Check sheet for the modelled part. Datum: model origin and axes. Units: mm. A direction names the side the tool comes from. Round coordinates to 2 decimals unless told otherwise and drop trailing zeros. Loops run counter-clockwise (first coordinate to the right, second up) from the corner with the lowest first, then second, coordinate; pieces in that order, holes last. Notation, with made-up numbers: (-24, 81) -> (-10, 81) arc R16 ccw to (-10, 87) -> close; hole circle Ø2 at (40, 53.25). An arc over 180 degrees is marked (long way). One line per question, with ' | ' between items.
```python
from build123d import *

# Parameters (mm, degrees)
BASE_EXTRUDE_DEPTH = 3


with BuildPart() as part:
    # Sketch1 → Base-Extrude (new body)
    with BuildSketch(Plane.XY):
        with BuildLine():
            Line((457.287518249, -79.214649933), (453.745445311, -79.230530857))
            ThreePointArc((453.745445311, -79.230530857), (449.646042877, -88.708611573), (453.753998991, -98.182988118))
            Line((453.753998991, -98.182988118), (469.771556658, -98.182988118))
            Line((469.771556658, -98.182988118), (469.765330169, -116.15983969))
            Line((469.765330169, -116.15983969), (483.771556658, -116.15983969))
            Line((483.771556658, -116.15983969), (483.771556658, -98.182988118))
            Line((483.771556658, -98.182988118), (485.771556658, -98.182988118))
            Line((485.771556658, -98.182988118), (485.434474546, -91.751078274))
            Line((485.434474546, -91.751078274), (488.434474546, -91.751078274))
            Line((488.434474546, -91.751078274), (488.771556658, -98.182988118))
            Line((488.771556658, -98.182988118), (499.789114325, -98.182988118))
            ThreePointArc((499.789114325, -98.182988118), (503.897070438, -88.708611573), (499.797668004, -79.230530857))
            Line((499.797668004, -79.230530857), (496.255595066, -79.214649933))
            Line((496.255595066, -79.214649933), (496.255595066, -91.387236838))
            Line((496.255595066, -91.387236838), (493.156556658, -91.387236838))
            Line((493.156556658, -91.387236838), (493.156556658, -81.698972351))
            Line((493.156556658, -81.698972351), (460.386556658, -81.698972351))
            Line((460.386556658, -81.698972351), (460.386556658, -91.387236838))
            Line((460.386556658, -91.387236838), (457.287518249, -91.387236838))
            Line((457.287518249, -91.387236838), (457.287518249, -79.214649933))
        make_face()
    extrude(amount=BASE_EXTRUDE_DEPTH)


solid = part.part
```
(1) Mould release check, pull along Y, two halves, no side actions. Record for faces 1 (the face through (485, -98.183, 1)), 2 (the face through (483.772, -107, 1)), 3 (the face through (485.605, -95.012, 1.479)): +Y half, -Y half, draft (parallel to the pull), parting line (faces both ways), or undercut.
Answer:
face 1: -Y half | face 2: draft | face 3: undercut
(2) Sectioned sample at B-B, the plane y = -90. Record the cut outline in (x, z), and give its area (3 significant figures).
Answer:
outline: (449.71, 0) -> (457.29, 0) -> (457.29, 3) -> (449.71, 3) -> close; (460.39, 0) -> (493.16, 0) -> (493.16, 3) -> (460.39, 3) -> close; (496.26, 0) -> (503.83, 0) -> (503.83, 3) -> (496.26, 3) -> close | area: 144 mm2
(3) Set-up check for faces 4 (the face through (488.6, -94.9, 1.5)), 5 (the face through (462, -98.183, 1)), 6 (the face through (477, -81.699, 1)), 7 (the face through (476, -97, 3)), 8 (the face through (476, -97, 0)): record each of +Z, -Z, +X, -X, +Y, -Y from which the full face is reachable in a straight line by a thin tool's end or side.
Answer:
face 4: +Z, -Z, -Y | face 5: +Z, -Z, -X, -Y | face 6: +Z, -Z, +Y | face 7: +Z, +X, -X, +Y, -Y | face 8: -Z, +X, -X, +Y, -Y
(4) Go/stop test with flat-tipped pins: pin 1 (0.9 mm diameter, centred on y = -88, z = 1.5, fed in from +X); pin 2 (1 mm diameter, centred on y = -96, z = 2.5, fed in from -X); pin 3 (5 mm diameter, centred on x = 496.5, y = -101.5, fed in from -Z); pin 4 (0.9 mm diameter, centred on x = 487, z = 1, fed in from -Y). Record where each tip stops, or that it passes through.
Answer:
pin 1: stops at x = 503.89 | pin 2: stops at x = 451.57 | pin 3: passes through | pin 4: stops at y = -91.75
(5) Scan lines: probe 1 along X at (y, z) = (-82, 2.3); probe 2 along X at (y, z) = (-85, 2.15); probe 3 along Y at (x, z) = (467, 2.6). Record each from-to range of solid material in increasing order.
Answer:
probe 1: x = 451.51 to 457.29, 460.39 to 493.16, 496.26 to 502.03 | probe 2: x = 450.18 to 457.29, 460.39 to 493.16, 496.26 to 503.36 | probe 3: y = -98.18 to -81.7
(6) Sectioned sample at C-C, the plane y = -96. Record the cut outline in (x, z), and give its area (3 significant figures).
Answer:
outline: (451.89, 0) -> (485.66, 0) -> (485.66, 3) -> (451.89, 3) -> close; (488.66, 0) -> (501.65, 0) -> (501.65, 3) -> (488.66, 3) -> close | area: 140 mm2
(7) Sectioned sample at A-A, the plane z = 0.55. Record the cut outline in (x, y).
Answer:
outline: (453.75, -98.18) -> (469.77, -98.18) -> (469.77, -116.16) -> (483.77, -116.16) -> (483.77, -98.18) -> (485.77, -98.18) -> (485.43, -91.75) -> (488.43, -91.75) -> (488.77, -98.18) -> (499.79, -98.18) arc R12.99 ccw to (499.8, -79.23) -> (496.26, -79.21) -> (496.26, -91.39) -> (493.16, -91.39) -> (493.16, -81.7) -> (460.39, -81.7) -> (460.39, -91.39) -> (457.29, -91.39) -> (457.29, -79.21) -> (453.75, -79.23) arc R12.99 ccw to start
(8) Sectioned sample at D-D, the plane x = 468. Record the cut outline in (y, z).
Answer:
outline: (-98.18, 0) -> (-81.7, 0) -> (-81.7, 3) -> (-98.18, 3) -> close
